Geometry: final body of the model. Coordinates: model frame, mm. Face numbers are marked on the shaded views. A direction names the side the tool comes from. Coordinates: 2 decimals unless noted, no trailing zeros. Write each loop counter-clockwise with the first axis right and the second up, starting at its lowest first coordinate (ties: lowest second). Pieces come first, ordered by that corner, then holes. Notation, with made-up numbers: (79, 77.5) -> (129, 77.5) arc R30 ccw to (129, 102.5) -> close; hole circle Ø1 at (-34, 27.5). An arc over 180 degrees is marked (long way). One line per item, written item: value.
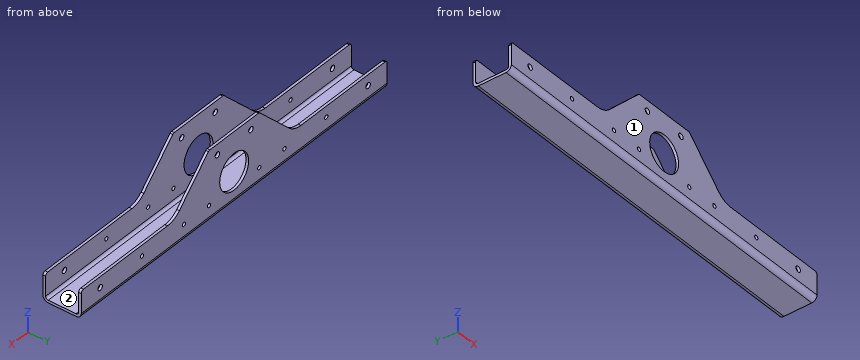
```python
from build123d import *

# Parameters (mm, degrees)
BASE_FLANGE1_DEPTH = 463.55
SKETCH6_R          = 21.9075
CUT_EXTRUDE1_DEPTH = 474.696057033
CUT_EXTRUDE2_DEPTH = 474.696057033
SKETCH8_R          = 3.3782
SKETCH8_R_2        = 2.4257
CUT_EXTRUDE3_DEPTH = 474.696057033
SKETCH9_R          = 3.3782
CUT_EXTRUDE4_DEPTH = 474.696057033
FILLET1_R          = 25.4
FILLET2_R          = 3.175


# Sheet-metal steps are written as plain solids
with BuildPart() as part:
    # Sketch1 → Base-Flange1 (new body)
    with BuildSketch(Plane(origin=(0, 0, 0), x_dir=(0, 0, -1), z_dir=(1, 0, 0))):
        with BuildLine():
            Line((0, 0), (79.375, 0))
            ThreePointArc((79.375, 0), (81.62006403, 0.92993597), (82.55, 3.175))
            Line((82.55, 3.175), (82.55, 36.957))
            ThreePointArc((82.55, 36.957), (81.62006403, 39.20206403), (79.375, 40.132))
            Line((79.375, 40.132), (0, 40.132))
            Line((0, 40.132), (0, 43.307))
            Line((0, 43.307), (79.375, 43.307))
            ThreePointArc((79.375, 43.307), (83.865128061, 41.447128061), (85.725, 36.957))
            Line((85.725, 36.957), (85.725, 3.175))
            ThreePointArc((85.725, 3.175), (83.865128061, -1.315128061), (79.375, -3.175))
            Line((79.375, -3.175), (0, -3.175))
            Line((0, -3.175), (0, 0))
        make_face()
    extrude(amount=BASE_FLANGE1_DEPTH)

    # Sketch6 → Cut-Extrude1 (cut, through all)
    with BuildSketch(Plane(origin=(0, 43.307, 0), x_dir=(1, 0, 0), z_dir=(0, 1, 0))):
        with Locations(Location((231.775, 47.625, 0), (0, 0, 270))):
            Circle(SKETCH6_R)
    extrude(amount=-CUT_EXTRUDE1_DEPTH, mode=Mode.SUBTRACT)

    # Sketch7 → Cut-Extrude2 (cut, through all)
    with BuildSketch(Plane(origin=(0, 43.307, 0), x_dir=(1, 0, 0), z_dir=(0, 1, 0))):
        Polygon((141.2748, 52.4002), (0, 52.4002), (0, 0), (193.675, 0), align=None)
        Polygon((322.2752, 52.4002), (269.875, 0), (463.55, 0), (463.55, 52.4002), align=None)
    extrude(amount=-CUT_EXTRUDE2_DEPTH, mode=Mode.SUBTRACT)

    # Sketch8 → Cut-Extrude3 (cut, through all)
    with BuildSketch(Plane(origin=(0, 43.307, 0), x_dir=(1, 0, 0), z_dir=(0, 1, 0))):
        with Locations(Location((28.575, 65.405, 0), (0, 0, 270))):
            Circle(SKETCH8_R)
        with Locations(Location((92.075, 65.405, 0), (0, 0, 270))):
            Circle(SKETCH8_R_2)
        with Locations(Location((193.675, 65.405, 0), (0, 0, 270))):
            Circle(SKETCH8_R_2)
        with Locations(Location((269.875, 65.405, 0), (0, 0, 270))):
            Circle(SKETCH8_R_2)
        with Locations(Location((371.475, 65.405, 0), (0, 0, 270))):
            Circle(SKETCH8_R_2)
        with Locations(Location((434.975, 65.405, 0), (0, 0, 270))):
            Circle(SKETCH8_R)
        with Locations(Location((155.575, 65.405, 0), (0, 0, 270))):
            Circle(SKETCH8_R_2)
        with Locations(Location((307.975, 65.405, 0), (0, 0, 270))):
            Circle(SKETCH8_R_2)
    extrude(amount=-CUT_EXTRUDE3_DEPTH, mode=Mode.SUBTRACT)

    # Sketch9 → Cut-Extrude4 (cut, through all)
    with BuildSketch(Plane(origin=(0, 43.307, 0), x_dir=(1, 0, 0), z_dir=(0, 1, 0))):
        with Locations(Location((257.175, 12.7, 0), (0, 0, 270))):
            Circle(SKETCH9_R)
        with Locations(Location((206.375, 12.7, 0), (0, 0, 270))):
            Circle(SKETCH9_R)
    extrude(amount=-CUT_EXTRUDE4_DEPTH, mode=Mode.SUBTRACT)

    # Fillet1
    fillet1_edges = [part.edges().sort_by_distance(p)[0] for p in [
        (141.2748, 41.7195, -52.4002),
        (141.2748, -1.5875, -52.4002),
        (322.2752, 41.7195, -52.4002),
        (322.2752, -1.5875, -52.4002),
    ]]
    fillet(fillet1_edges, radius=FILLET1_R)

    # Fillet2
    fillet2_edges = [part.edges().sort_by_distance(p)[0] for p in [
        (0, 41.7195, -52.4002),
        (193.675, 41.7195, 0),
        (193.675, -1.5875, 0),
        (0, -1.5875, -52.4002),
        (463.55, 41.7195, -52.4002),
        (269.875, 41.7195, 0),
        (463.55, -1.5875, -52.4002),
        (269.875, -1.5875, 0),
    ]]
    fillet(fillet2_edges, radius=FILLET2_R)


solid = part.part
```
(1) Section C-C (x = 404.5). Return the cut outline in (y, z) (3 decimals), then the cut area to 3 significant figures.
Responses:
outline: (-3.175, -79.375) arc R6.35 ccw to (3.175, -85.725) -> (36.957, -85.725) arc R6.35 ccw to (43.307, -79.375) -> (43.307, -52.4) -> (40.132, -52.4) -> (40.132, -79.375) arc R3.175 cw to (36.957, -82.55) -> (3.175, -82.55) arc R3.175 cw to (0, -79.375) -> (0, -52.4) -> (-3.175, -52.4) -> close
area: 326 mm2
(2) Section A-A (z = -36.5). Return the cut outline in (x, y) (3 decimals), then the cut area to 3 significant figures.
Responses:
outline: (157.175, -3.175) -> (212.902, -3.175) -> (212.902, 0) -> (157.175, 0) -> close; (157.175, 40.132) -> (212.902, 40.132) -> (212.902, 43.307) -> (157.175, 43.307) -> close; (250.648, -3.175) -> (306.375, -3.175) -> (306.375, 0) -> (250.648, 0) -> close; (250.648, 40.132) -> (306.375, 40.132) -> (306.375, 43.307) -> (250.648, 43.307) -> close
area: 708 mm2
(3) Section D-D (y = 12). Return the cut outline in (x, z) (3 decimals), then the cut area to 3 significant figures.
Responses:
outline: (0, -85.725) -> (463.55, -85.725) -> (463.55, -82.55) -> (0, -82.55) -> close
area: 1,470 mm2
(4) Line query: line 1 (Y direction, x = 283.5, z = -62.5) (3 decimals); line 2 (X direction, y = 41.8, z = -12.7) (3 decimals); line 3 (Z direction, x = 327, y = 9) (3 decimals). Output: solid intervals per line, ascending. Write a range as [from, to].
Responses:
line 1: y = [-3.175, 0], [40.132, 43.307]
line 2: x = [180.975, 202.997], [209.753, 253.797], [260.553, 282.575]
line 3: z = [-85.725, -82.55]
(5) First-contact query: pin 1 (4 mm diameter, centred on x = 257.175, z = -12.7, fed in from -Y) (3 decimals); pin 2 (1 mm diameter, centred on x = 55.5, y = -1.5, fed in from +Z); pin 3 (5 mm diameter, centred on x = 257.5, y = 8.5, fed in from +Z). Flat tips, straight axial feed; report the tip coordinate or a pass-through.
Responses:
pin 1: passes through
pin 2: stops at z = -52.4
pin 3: stops at z = -82.55
(6) Reachability of the marked faces 1 and 2 from +Z, -Z, +X, -X, +Y, -Y: full face, straight path, thin tool, end or side. Return the list, or none.
Responses:
face 1: +Z, -Z, +X, -X, -Y
face 2: +Z, +X, -X
(7) Section B-B (x = 243). Return the cut outline in (y, z) (3 decimals), then the cut area to 3 significant figures.
Responses:
outline: (-3.175, -79.375) arc R6.35 ccw to (3.175, -85.725) -> (36.957, -85.725) arc R6.35 ccw to (43.307, -79.375) -> (43.307, -66.438) -> (40.132, -66.438) -> (40.132, -79.375) arc R3.175 cw to (36.957, -82.55) -> (3.175, -82.55) arc R3.175 cw to (0, -79.375) -> (0, -66.438) -> (-3.175, -66.438) -> close; (-3.175, -28.812) -> (0, -28.812) -> (0, 0) -> (-3.175, 0) -> close; (40.132, -28.812) -> (43.307, -28.812) -> (43.307, 0) -> (40.132, 0) -> close
area: 420 mm2
